The listing builds one solid part. Answer for the finished solid, in the listing's coordinates (mm). Face numbers are marked on the shaded views. A direction names the side the tool comes from. Coordinates: 2 decimals unless noted, no trailing zeros. Loops run counter-clockwise (first coordinate to the right, second up) from the corner with the lowest first, then second, coordinate; pieces in that order, holes last. Notation, with made-up numbers: (-31.5, 50) - (16.5, 50) arc R18 ccw to (16.5, 55) - close; hole circle Ø11 at (15, -26). An arc over 180 degrees is marked (long way). Use one line per item in the form item = value. Start each with the question number.
```python
from build123d import *

# Parameters (mm, degrees)
ESQUISSE1_W        = 20
ESQUISSE1_H        = 40.3
BOSS_EXTRU_1_DEPTH = 36.1
ESQUISSE3_W        = 19.8
ESQUISSE3_H        = 2
BOSS_EXTRU_3_DEPTH = 7.6
ESQUISSE5_W        = 19.8
ESQUISSE5_H        = 2
BOSS_EXTRU_4_DEPTH = 7.6
ESQUISSE6_R        = 4
BOSS_EXTRU_5_DEPTH = 8


with BuildPart() as part:
    # Esquisse1 → Boss.-Extru.1 (new body)
    with BuildSketch(Plane.XY):
        Rectangle(ESQUISSE1_W, ESQUISSE1_H)
    extrude(amount=BOSS_EXTRU_1_DEPTH)

    # Esquisse3 → Boss.-Extru.3 (add)
    with BuildSketch(Plane(origin=(-10, -20.15, 0), x_dir=(1, 0, 0), z_dir=(0, -1, 0))):
        with Locations((10, 8.5)):
            Rectangle(ESQUISSE3_W, ESQUISSE3_H)
    extrude(amount=BOSS_EXTRU_3_DEPTH)

    # Esquisse5 → Boss.-Extru.4 (add)
    with BuildSketch(Plane(origin=(0, 20.15, 0), x_dir=(1, 0, 0), z_dir=(0, 1, 0))):
        with Locations((0, -8.5)):
            Rectangle(ESQUISSE5_W, ESQUISSE5_H)
    extrude(amount=BOSS_EXTRU_4_DEPTH)

    # Esquisse6 → Boss.-Extru.5 (add)
    with BuildSketch(Plane(origin=(0, 0, 0), x_dir=(-1, 0, 0), z_dir=(0, 0, -1))):
        with Locations(Location((0, -13.5, 0), (0, 0, 180))):  # turned: the seam where the file's is
            Circle(ESQUISSE6_R)
    extrude(amount=BOSS_EXTRU_5_DEPTH)


solid = part.part
```
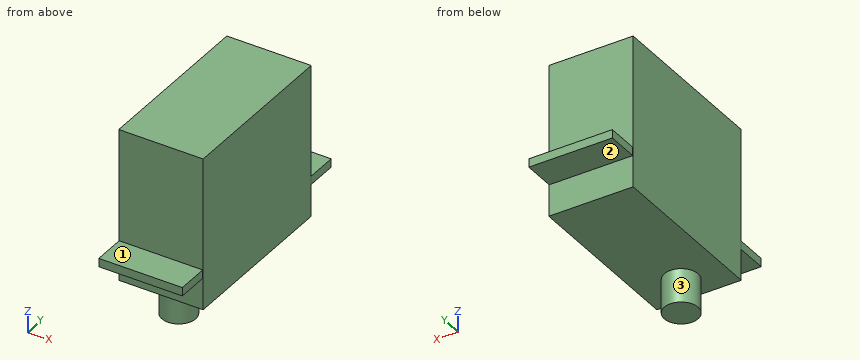
(1) A cutting plane is placed at A-A (x = 0). Determine the outline of the cut face in (y, z).
(2) Find the intervals of material crossed by probe 1 along Z at (x, y) = (7.25, 24.5); probe 2 along Z at (x, y) = (6.75, -5); probe 3 along Y at (x, z) = (4.25, 22.5), in increasing order. Write a range as from..to.
(3) A cutting plane is placed at C-C (x = -4.75). Determine the outline of the cut face in (y, z), then the cut area to 3 significant figures.
(4) A cutting plane is placed at D-D (z = 3.5). Determine the outline of the cut face in (x, y), then the cut area to 3 significant figures.
(5) For the marked faces 1, 2 and 3, determine the directions among +Z, -Z, +X, -X, +Y, -Y from which every point of the face is accessible in a straight line to the end or side of a thin tool.
(6) A cutting plane is placed at B-B (y = -13.5). Determine the outline of the cut face in (x, z).
(7) Each of these flat-tipped pins is pushed along its axis until it touches: pin 1 Ø2 at (x, z) = (7.5, 12) entering from -Y; pin 2 Ø6 at (x, y) = (-4.5, 23.5) entering from +Z; pin 3 Ø2 at (x, y) = (2, -19) entering from -Z. Where does it stop, or does it pass through?
Evaluation:
q1.outline = (-27.75, 7.5) - (-20.15, 7.5) - (-20.15, 0) - (-17.5, 0) - (-17.5, -8) - (-9.5, -8) - (-9.5, 0) - (20.15, 0) - (20.15, 7.5) - (27.75, 7.5) - (27.75, 9.5) - (20.15, 9.5) - (20.15, 36.1) - (-20.15, 36.1) - (-20.15, 9.5) - (-27.75, 9.5) - close
q2.probe_1 = 7.5..9.5
q2.probe_2 = 0..36.1
q2.probe_3 = -20.15..20.15
q3.outline = (-27.75, 7.5) - (-20.15, 7.5) - (-20.15, 0) - (20.15, 0) - (20.15, 7.5) - (27.75, 7.5) - (27.75, 9.5) - (20.15, 9.5) - (20.15, 36.1) - (-20.15, 36.1) - (-20.15, 9.5) - (-27.75, 9.5) - close
q3.area = 1,490 mm^2
q4.outline = (-10, -20.15) - (10, -20.15) - (10, 20.15) - (-10, 20.15) - close
q4.area = 806 mm^2
q5.face_1 = +Z, +X, -X, -Y
q5.face_2 = -Z, +X, -X, +Y
q5.face_3 = -Z
q6.outline = (-10, 0) - (-4, 0) - (-4, -8) - (4, -8) - (4, 0) - (10, 0) - (10, 36.1) - (-10, 36.1) - close
q7.pin_1 = -20.15
q7.pin_2 = 9.5
q7.pin_3 = 0
